Geometry: see drawing. Coordinates: mm, zero at the bounding-box minimum. A direction names the side the tool comes from. Round coordinates to 2 decimals unless told otherwise and drop trailing zeros. Return JSON: item names as keys, results as strings. Group by question number.
1. Section A-A on y = 6. Count the separate pieces of the cut face and the enclosed holes in it, and give its area (3 significant figures).
2. Draft query along X for the marked faces 1, 2 and 3. Return one class per face: +X half, -X half, draft (parallel to the pull), parting line (faces both ways), or undercut.
3. First-contact query: pin 1 Ø6 at (x, z) = (72.5, 11) entering from +Y; pin 2 Ø2 at (x, z) = (65, 65.5) entering from -Y; pin 3 Ø5 at (x, z) = (73.025, 9.525) entering from +Y; pin 4 Ø2 at (y, z) = (8.5, 10) entering from -X (1 decimal). Flat tips, straight axial feed; report the tip coordinate or a pass-through.
4. Material intervals for probe 1 along X at (y, z) = (6.75, 35.5); probe 2 along Z at (x, y) = (57, 9.75); probe 3 along Y at (x, z) = (75, 18), sorted ascending.
5. Set-up query: the marked faces 4 and 5. Return all of +Z, -Z, +X, -X, +Y, -Y with unobstructed straight access to the full face (end or side cutting, diameter ignored); none if empty.
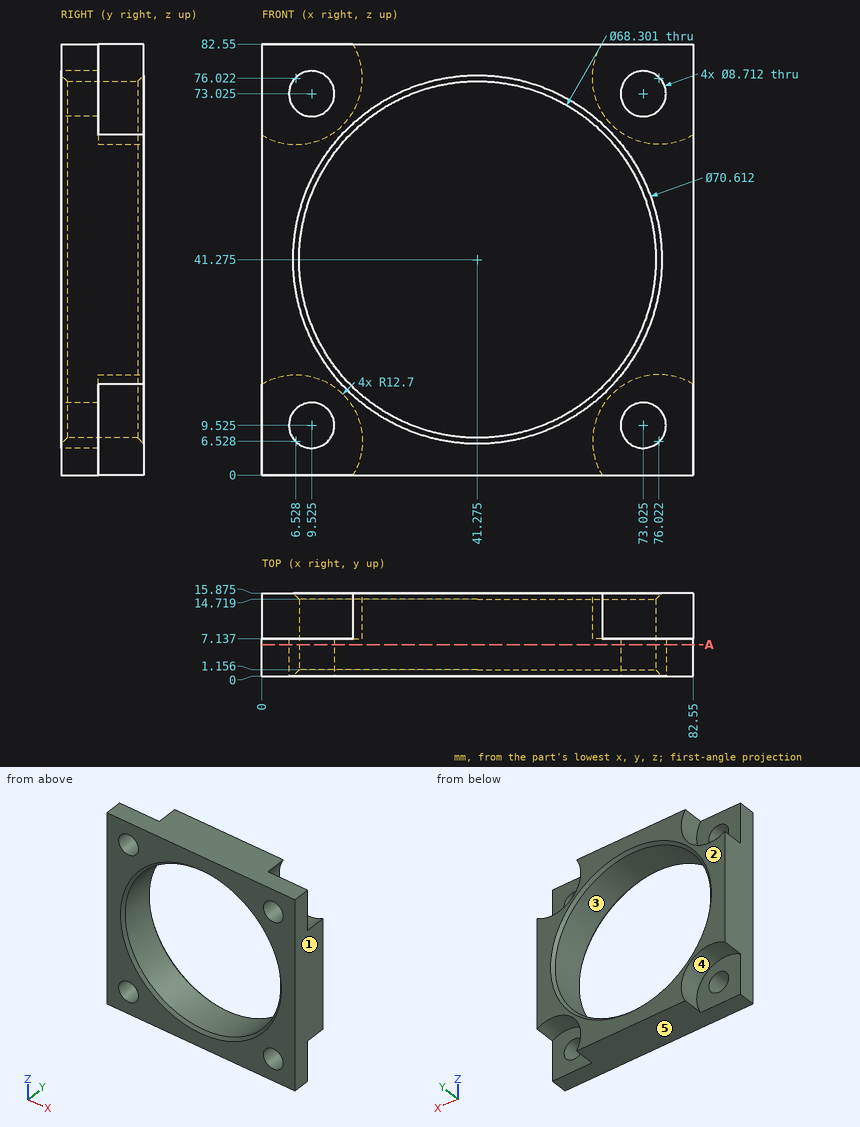
Taken from the geometry:
{
 "1": {"separate pieces": "1", "enclosed holes": "5", "area": "2,910 mm2"},
 "2": {"face 1": "+X half", "face 2": "draft", "face 3": "undercut"},
 "3": {"pin 1": "y = 7.14", "pin 2": "y = 0.4", "pin 3": "through", "pin 4": "x = 18.4"},
 "4": {"probe 1": "0 to 7.62, 74.93 to 82.55", "probe 2": "0 to 10.96, 71.59 to 82.55", "probe 3": "0 to 7.14"},
 "5": {"face 4": "+Y", "face 5": "-Z, +X, -X, +Y, -Y"}
}
